Autodesk Fusion 360 part; units mm, degrees
sketch "Plate" plane through (0, 0, 0) normal (0, 1, 0) x (1, 0, 0)
  line L0 (0, 0) -> (7, 0)
  line L1 (7, 0) -> (7, -74)
  line L2 (7, -74) -> (0, -74)
  line L3 (0, -74) -> (0, 0)
  dimension "d58" = 7
  dimension "d59" = 74
extrude "Plate (1)" add sketch "Plate" along normal mid plane 24
sketch "Hook profile" plane through (0, 0, 0) normal (0, 1, 0) x (1, 0, 0)
  line L0 (0, -72) -> (-8.3, -72)
  line L1 (-8.3, -72) -> (-8.3, -55)
  line L2 (-8.3, -55) -> (-5.3, -55)
  line L3 (-5.3, -55) -> (-3.8, -56.5)
  line L4 (-3.8, -56.5) -> (-3.8, -67)
  line L5 (-3.8, -67) -> (0, -67)
  line L6 (0, -67) -> (0, -72)
  dimension "d62" = 72
  dimension "d63" = 8.3
  dimension "d64" = 3.8
  dimension "d65" = 5
  dimension "d66" = 10.5
  dimension "d67" = 1.5
  dimension "d68" = 1.5
extrude "Hook profile (1)" add sketch "Hook profile" along normal mid plane 2.4
pattern_linear "Hook rows" count 2 spacing 25.4 along (0, 0, -1) count 3 spacing 0 along (0, 0, 1) of "Hook profile (1)"
sketch "Nut track 0" plane through (0, 0, 0) normal (0, 1, 0) x (1, 0, 0)
  line L0 (0, -53.545) -> (6, -53.545)
  line L1 (6, -53.545) -> (6, -65.055)
  line L2 (6, -65.055) -> (0, -65.055)
  line L3 (0, -65.055) -> (0, -53.545)
  line L4 (0, -1.75) -> (0, -22.5)
  dimension "d75" = 53.545
  dimension "d76" = 6
  dimension "d77" = 65.055
extrude "Nut track 0 (1)" cut sketch "Nut track 0" along normal mid plane 34
sketch "Bolt slot 0" plane through (0, 0, 0) normal (0, 1, 0) x (1, 0, 0)
  line L0 (0, -55.8) -> (8, -55.8)
  line L1 (8, -55.8) -> (8, -62.8)
  line L2 (8, -62.8) -> (0, -62.8)
  line L3 (0, -62.8) -> (0, -55.8)
  line L4 (0, -1.75) -> (0, -22.5)
  dimension "d80" = 55.8
  dimension "d81" = 8
  dimension "d82" = 62.8
extrude "Bolt slot 0 (1)" cut sketch "Bolt slot 0" along normal mid plane 14
sketch "Nut track 1" plane through (0, 0, 0) normal (0, 1, 0) x (1, 0, 0)
  line L0 (0, -28.145) -> (6, -28.145)
  line L1 (6, -28.145) -> (6, -39.655)
  line L2 (6, -39.655) -> (0, -39.655)
  line L3 (0, -39.655) -> (0, -28.145)
  line L4 (0, -1.75) -> (0, -22.5)
  dimension "d85" = 28.145
  dimension "d86" = 6
  dimension "d87" = 39.655
extrude "Nut track 1 (1)" cut sketch "Nut track 1" along normal mid plane 34
sketch "Bolt slot 1" plane through (0, 0, 0) normal (0, 1, 0) x (1, 0, 0)
  line L0 (0, -30.4) -> (8, -30.4)
  line L1 (8, -30.4) -> (8, -37.4)
  line L2 (8, -37.4) -> (0, -37.4)
  line L3 (0, -37.4) -> (0, -30.4)
  line L4 (0, -1.75) -> (0, -22.5)
  dimension "d90" = 30.4
  dimension "d91" = 8
  dimension "d92" = 37.4
extrude "Bolt slot 1 (1)" cut sketch "Bolt slot 1" along normal mid plane 14
equation "bracketWidth = 24.0 mm"
equation "hookTabWidth = slotWidth - 0.8 mm"
equation "slotPitchVertical = 25.4 mm"
equation "faceMetalThickness = 2.0 mm"
equation "hookThroat = faceMetalThickness + 1.8 mm"
equation "hookNeckHeight = 5.0 mm"
equation "hookLipThickness = 4.5 mm"
equation "hookLipDrop = 12.0 mm"
equation "hookLipChamfer = 1.5 mm"
equation "topHookNeckTop = 72.0 mm"
equation "plateThickness = 7.0 mm"
equation "plateHeight = 74.0 mm"
equation "boltSlotHeight = 7.0 mm"
equation "boltSlotLength = 14.0 mm"
equation "nutTrackHeight = 11.51 mm"
equation "nutTrackDepth = 6.0 mm"
equation "slotWidth = 3.2 mm"
equation "topBoltCentre = 59.3 mm"
equation "d58 = plateThickness"
equation "d59 = plateHeight"
equation "d60 = bracketWidth"
equation "d62 = topHookNeckTop"
equation "d63 = hookThroat + hookLipThickness"
equation "d64 = hookThroat"
equation "d65 = hookNeckHeight"
equation "d66 = hookLipDrop - hookLipChamfer"
equation "d67 = hookLipChamfer"
equation "d68 = hookLipChamfer"
equation "d69 = hookTabWidth"
equation "d75 = topBoltCentre - nutTrackHeight / 2"
equation "d76 = nutTrackDepth"
equation "d77 = topBoltCentre + nutTrackHeight / 2"
equation "d78 = bracketWidth + 10 mm"
equation "d80 = topBoltCentre - boltSlotHeight / 2"
equation "d81 = plateThickness + 1 mm"
equation "d82 = topBoltCentre + boltSlotHeight / 2"
equation "d83 = boltSlotLength"
equation "d85 = topBoltCentre - 1 * slotPitchVertical - nutTrackHeight / 2"
equation "d86 = nutTrackDepth"
equation "d87 = topBoltCentre - 1 * slotPitchVertical + nutTrackHeight / 2"
equation "d88 = bracketWidth + 10 mm"
equation "d90 = topBoltCentre - 1 * slotPitchVertical - boltSlotHeight / 2"
equation "d91 = plateThickness + 1 mm"
equation "d92 = topBoltCentre - 1 * slotPitchVertical + boltSlotHeight / 2"
equation "d93 = boltSlotLength"
Input: part model. Units: mm. Frame: model coordinates. A direction names the side the tool comes from. Round coordinates to 2 decimals unless told otherwise and drop trailing zeros. Loops run counter-clockwise (first coordinate to the right, second up) from the corner with the lowest first, then second, coordinate; pieces in that order, holes last.
1) Pin query (flat end, axial travel): pin 1 (1.5 mm diameter, centred on x = -5.5, z = 60.5, fed in from -Y); pin 2 (1 mm diameter, centred on x = 5, z = 34, fed in from +Y); pin 3 (2 mm diameter, centred on x = -5.5, y = -1.5, fed in from -Z); pin 4 (0.7 mm diameter, centred on x = -2.5, y = 0, fed in from -Z). Return the tip coordinate at first contact, or that it passes through.
Ans:
pin 1: stops at y = -1.2
pin 2: passes through
pin 3: stops at z = 29.6
pin 4: stops at z = 41.6
2) Set-up query: faces 1 (the flat face through (-2, 0, 41.6)), 2 (the flat face through (-5, 1.2, 65)), 3 (the flat face through (-7, 0, 29.6)), 4 (the flat face through (-5, -1.2, 65)). Return all of +Z, -Z, +X, -X, +Y, -Y with unobstructed straight access to the full face (end or side cutting, diameter ignored); none if empty.
Ans:
face 1: -Z, +Y, -Y
face 2: +Z, -Z, -X, +Y
face 3: -Z, -X, +Y, -Y
face 4: +Z, -Z, -X, -Y
3) Section query A-A on y = -3. Return the cut outline in (x, z) (3 decimals), plus the area to 3 significant figures.
Ans:
outline: (0, 0) - (7, 0) - (7, 30.4) - (6, 30.4) - (6, 28.145) - (0, 28.145) - close; (0, 39.655) - (6, 39.655) - (6, 37.4) - (7, 37.4) - (7, 55.8) - (6, 55.8) - (6, 53.545) - (0, 53.545) - close; (0, 65.055) - (6, 65.055) - (6, 62.8) - (7, 62.8) - (7, 74) - (0, 74) - close
area: 366 mm2
4) Section query D-D on x = -1.75. Return the cut outline in (y, z), plus the area to 3 significant figures.
Ans:
outline: (-1.2, 41.6) - (1.2, 41.6) - (1.2, 46.6) - (-1.2, 46.6) - close; (-1.2, 67) - (1.2, 67) - (1.2, 72) - (-1.2, 72) - close
area: 24.0 mm2
5) Material intervals for line 1 (Z direction, x = 5.75, y = 10) (3 decimals); line 2 (Y direction, x = -7, z = 38); line 3 (X direction, y = -5.5, z = 68), sorted ascending.
Ans:
line 1: z = 0 to 28.145, 39.655 to 53.545, 65.055 to 74
line 2: y = -1.2 to 1.2
line 3: x = 0 to 7
6) Section query C-C on x = 3. Return the cut outline in (y, z) (3 decimals).
Ans:
outline: (-12, 0) - (12, 0) - (12, 28.145) - (-12, 28.145) - close; (-12, 39.655) - (12, 39.655) - (12, 53.545) - (-12, 53.545) - close; (-12, 65.055) - (12, 65.055) - (12, 74) - (-12, 74) - close
7) Pull-direction query (Z, two-part tool) for faces 5 (the flat face through (-5, 1.2, 40)), 6 (the flat face through (-4, 0, 46.6)), 7 (the flat face through (4, 0, 74)); classes: released by +Z, released by -Z, zero draft, split by the parting line, or undercut.
Ans:
face 5: zero draft
face 6: undercut
face 7: released by +Z
8) Section query B-B on z = 32.5. Return the cut outline in (x, y), plus the area to 3 significant figures.
Ans:
outline: (-8.3, -1.2) - (-3.8, -1.2) - (-3.8, 1.2) - (-8.3, 1.2) - close; (6, -12) - (7, -12) - (7, -7) - (6, -7) - close; (6, 7) - (7, 7) - (7, 12) - (6, 12) - close
area: 20.8 mm2
